from build123d import *
from build123d.topology import SkipClean

# Parameters (mm, degrees)
BOSS_EXTRUDE1_DEPTH     = 1.4
BOSS_EXTRUDE2_DEPTH     = 0.7
SKETCH3_W               = 2
SKETCH3_H               = 1
SKETCH3_R               = 2.5
BOSS_EXTRUDE3_DEPTH     = 0.6
SKETCH4_R               = 2
SKETCH4_R_2             = 0.75
SKETCH4_W               = 2
SKETCH4_H               = 1
BOSS_EXTRUDE4_DEPTH     = 1.3
BOSS_EXTRUDE6_REACH     = 14
CHAMFER1_SIZE           = 2
SKETCH7_W               = 12.5
SKETCH7_H               = 6.503126956
BOSS_EXTRUDE7_DEPTH     = 7.75
SKETCH8_W               = 12.5
SKETCH8_H               = 7.5
BOSS_EXTRUDE8_DEPTH     = 10
FILLET1_R               = 3
SKETCH9_W               = 11
SKETCH9_H               = 1.9
BOSS_EXTRUDE9_DEPTH     = 3.003289
BOSS_EXTRUDE10_START    = -0.75
SKETCH10_R              = 0.75
SKETCH10_R_2            = 2
SKETCH10_W              = 2
SKETCH10_H              = 1
BOSS_EXTRUDE10_DEPTH    = 0.75
SKETCH11_R              = 2
BOSS_EXTRUDE11_DEPTH    = 2.5
FILLET2_SIZE            = 2.5
FILLET2_SIZE_2          = 1
CUT_EXTRUDE1_DEPTH      = 32.401632123
CUT_EXTRUDE1_DEPTH_BACK = 32.401632123
SKETCH12_R              = 0.75
CUT_EXTRUDE2_REACH      = 34.731
SKETCH13_W              = 2.1
SKETCH13_H              = 1


with BuildPart() as part:
    # Sketch1 → Boss-Extrude1 (new body)
    with BuildSketch(Plane.XY):
        with BuildLine():
            Line((-5.5, 5.809475019), (-5.5, -2.5))
            Line((-5.5, -2.5), (-2.5, -5.5))
            Line((-2.5, -5.5), (2.5, -5.5))
            Line((2.5, -5.5), (5.5, -2.5))
            Line((5.5, -2.5), (5.5, 5.809475019))
            ThreePointArc((5.5, 5.809475019), (0, -8), (-5.5, 5.809475019))
        make_face()
    extrude(amount=BOSS_EXTRUDE1_DEPTH)

    # Sketch2 → Boss-Extrude2 (add)
    with BuildSketch(Plane.XY.offset(1.4)):
        with BuildLine():
            Line((-1, -5.5), (-1, -6.5))
            Line((-1, -6.5), (1, -6.5))
            Line((1, -6.5), (1, -5.5))
            Line((1, -5.5), (2.5, -5.5))
            Line((2.5, -5.5), (5.5, -2.5))
            Line((5.5, -2.5), (5.5, 5.809475019))
            ThreePointArc((5.5, 5.809475019), (0, -8), (-5.5, 5.809475019))
            Line((-5.5, 5.809475019), (-5.5, -2.5))
            Line((-5.5, -2.5), (-2.5, -5.5))
            Line((-2.5, -5.5), (-1, -5.5))
        make_face()
    extrude(amount=BOSS_EXTRUDE2_DEPTH)

    # Sketch3 → Boss-Extrude3 (add)
    with BuildSketch(Plane.XY.offset(2.1)):
        with BuildLine():
            Line((-5.5, 6.5), (-5.5, 5.809475019))
            ThreePointArc((-5.5, 5.809475019), (0, -8), (5.5, 5.809475019))
            Line((5.5, 5.809475019), (5.5, 6.5))
            Line((5.5, 6.5), (-5.5, 6.5))
        make_face()
        with Locations((0, -6)):
            Rectangle(SKETCH3_W, SKETCH3_H, mode=Mode.SUBTRACT)
        Circle(SKETCH3_R, mode=Mode.SUBTRACT)
        with BuildLine():
            ThreePointArc((-3.499999999, 5.5), (-4.249999999, 4.75), (-4.999999999, 5.5))
            ThreePointArc((-4.999999999, 5.5), (-4.249999999, 6.25), (-3.499999999, 5.5))
        make_face(mode=Mode.SUBTRACT)
        with BuildLine():
            ThreePointArc((5.000000001, 5.5), (4.250000001, 4.75), (3.500000001, 5.5))
            ThreePointArc((3.500000001, 5.5), (4.250000001, 6.25), (5.000000001, 5.5))
        make_face(mode=Mode.SUBTRACT)
    extrude(amount=BOSS_EXTRUDE3_DEPTH)

    # Sketch4 → Boss-Extrude4 (add)
    with SkipClean():  # the faces are left unmerged after this step: merging them gives an invalid solid
        with BuildSketch(Plane.XY.offset(2.7)):
            with BuildLine():
                Line((-5.5, 5.809475019), (-5.5, 6.5))
                Line((-5.5, 6.5), (5.5, 6.5))
                Line((5.5, 6.5), (5.5, 5.809475019))
                ThreePointArc((5.5, 5.809475019), (0, -8), (-5.5, 5.809475019))
            make_face()
            Circle(SKETCH4_R, mode=Mode.SUBTRACT)
            with Locations((-4.249999999, 5.5)):
                Circle(SKETCH4_R_2, mode=Mode.SUBTRACT)
            with Locations((4.250000001, 5.5)):
                Circle(SKETCH4_R_2, mode=Mode.SUBTRACT)
            with Locations((0, -6)):
                Rectangle(SKETCH4_W, SKETCH4_H, mode=Mode.SUBTRACT)
        extrude(amount=BOSS_EXTRUDE4_DEPTH)

    # Boss-Extrude6: up to this face of the body (flat: up to its plane)
    boss_extrude6_end = Plane(part.part.faces().sort_by_distance((0, -7.784071771, 4))[0])
    # Sketch5 → Boss-Extrude6 (add, up to the picked face)
    with BuildSketch(Plane.XY, mode=Mode.PRIVATE) as boss_extrude6_sk1:
        with BuildLine():
            Line((-6.25, 4.993746089), (-6.25, 18))
            Line((-6.25, 18), (6.25, 18))
            Line((6.25, 18), (6.25, 4.993746089))
            ThreePointArc((6.25, 4.993746089), (5.88914072, 5.414611858), (5.5, 5.809475019))
            Line((5.5, 5.809475019), (5.5, 6.5))
            Line((5.5, 6.5), (4.249999999, 8.5))
            ThreePointArc((4.249999999, 8.5), (0, 9.503288904), (-4.249999999, 8.5))
            Line((-4.249999999, 8.5), (-5.5, 6.5))
            Line((-5.5, 6.5), (-5.5, 5.809475019))
            ThreePointArc((-5.5, 5.809475019), (-5.88914072, 5.414611858), (-6.25, 4.993746089))
        make_face()
    boss_extrude6_tool1 = split(extrude(boss_extrude6_sk1.sketch, amount=BOSS_EXTRUDE6_REACH, mode=Mode.PRIVATE), bisect_by=boss_extrude6_end, keep=Keep.BOTH, mode=Mode.PRIVATE)
    add(boss_extrude6_tool1.solids().sort_by(Axis((0, 13.103061, 0), (0, 0, 1)))[0])

    # Chamfer1
    chamfer1_edges = [part.edges().sort_by_distance(p)[0] for p in [
        (0, 9.503288904, 0),
    ]]
    chamfer(chamfer1_edges, length=CHAMFER1_SIZE)

    # Sketch7 → Boss-Extrude7 (add)
    with BuildSketch(Plane(origin=(0, 0, 0), x_dir=(-1, 0, 0), z_dir=(0, 0, -1))):
        with Locations((0, 14.748436522)):
            Rectangle(SKETCH7_W, SKETCH7_H)
    extrude(amount=BOSS_EXTRUDE7_DEPTH)

    # Sketch8 → Boss-Extrude8 (add)
    with SkipClean():  # the faces are left unmerged after this step: merging them gives an invalid solid
        with BuildSketch(Plane(origin=(0, 18, 0), x_dir=(1, 0, 0), z_dir=(0, 1, 0))):
            with Locations((0, 4)):
                Rectangle(SKETCH8_W, SKETCH8_H)
        extrude(amount=BOSS_EXTRUDE8_DEPTH)

    # Fillet1
    # the kernel refuses this fillet: 3 mm, written as the material it adds along each edge
    with BuildSketch(Plane(origin=(-6.25, 18, -0.25), x_dir=(0, 0, 1), z_dir=(1, 0, 0))) as fillet1_piece_1:
        with BuildLine():
            CenterArc((FILLET1_R, -FILLET1_R), FILLET1_R, 90, 90)
            Line((0, -FILLET1_R), (0, 0))
            Line((0, 0), (FILLET1_R, 0))
        make_face()
    extrude(amount=12.5)

    # Sketch9 → Boss-Extrude9 (add)
    with BuildSketch(Plane(origin=(0, 6.5, 0), x_dir=(1, 0, 0), z_dir=(0, 1, 0))):
        with Locations((0, -3.05)):
            Rectangle(SKETCH9_W, SKETCH9_H)
    extrude(amount=BOSS_EXTRUDE9_DEPTH)

    # Sketch10 → Boss-Extrude10 (add)
    with SkipClean():  # the faces are left unmerged after this step: merging them gives an invalid solid
        with BuildSketch(Plane.XY.offset(4).offset(BOSS_EXTRUDE10_START)):
            with Locations((4.250000001, 5.5)):
                Circle(SKETCH10_R)
            with Locations((-4.249999999, 5.5)):
                Circle(SKETCH10_R)
            Circle(SKETCH10_R_2)
            with Locations((0, -6)):
                Rectangle(SKETCH10_W, SKETCH10_H)
        extrude(amount=BOSS_EXTRUDE10_DEPTH)
    add(part.part.scale(1), mode=Mode.REPLACE)  # the faces are merged on a copy

    # Sketch11 → Boss-Extrude11 (add)
    with BuildSketch(Plane(origin=(0, 0, -7.75), x_dir=(-1, 0, 0), z_dir=(0, 0, -1))):
        with Locations(Location((0, 15.622654783, 0), (0, 0, 180))):
            Circle(SKETCH11_R)
        with Locations(Location((0, 23.874218261, 0), (0, 0, 180))):
            Circle(SKETCH11_R)
    extrude(amount=BOSS_EXTRUDE11_DEPTH)

    # Fillet2
    # an asymmetric fillet: 2.5, 1 mm, written as the material it takes off along each edge
    with BuildSketch(Plane(origin=(0, 15.622654783, -10.25), x_dir=(1, 0, 0), z_dir=(0, 1, 0))) as fillet2_piece_1:
        with BuildLine():
            Bezier((2, -FILLET2_SIZE), (2, 0), (2 - FILLET2_SIZE_2, 0), weights=[1, 0.707106781, 1])
            Line((2 - FILLET2_SIZE_2, 0), (2, 0))
            Line((2, 0), (2, -FILLET2_SIZE))
        make_face()
    revolve(axis=Axis((0, 15.622654783, -10.25), (0, 0, -1)), mode=Mode.SUBTRACT)
    with BuildSketch(Plane(origin=(0, 23.874218261, -10.25), x_dir=(1, 0, 0), z_dir=(0, 1, 0))) as fillet2_piece_2:
        with BuildLine():
            Bezier((2, -FILLET2_SIZE), (2, 0), (2 - FILLET2_SIZE_2, 0), weights=[1, 0.707106781, 1])
            Line((2 - FILLET2_SIZE_2, 0), (2, 0))
            Line((2, 0), (2, -FILLET2_SIZE))
        make_face()
    revolve(axis=Axis((0, 23.874218261, -10.25), (0, 0, -1)), mode=Mode.SUBTRACT)

    # Sketch12 → Cut-Extrude1 (cut, two sides: drawn at the far end of the back side and taken through both)
    with BuildSketch(Plane(origin=(0, 0, -7.75), x_dir=(-1, 0, 0), z_dir=(0, 0, -1)).offset(-CUT_EXTRUDE1_DEPTH_BACK)):
        with Locations((-4.25, 15.7375)):
            Circle(SKETCH12_R)
        with Locations((-4.25, 23.9125)):
            Circle(SKETCH12_R)
        with Locations((4.25, 23.9125)):
            Circle(SKETCH12_R)
        with Locations((4.25, 15.7375)):
            Circle(SKETCH12_R)
    extrude(amount=CUT_EXTRUDE1_DEPTH + CUT_EXTRUDE1_DEPTH_BACK, mode=Mode.SUBTRACT)

    # Cut-Extrude2: up to this face of the body (flat: up to its plane)
    cut_extrude2_end = Plane(part.part.faces().sort_by_distance((-5.5, 2, 1.05))[0])
    # Sketch13 → Cut-Extrude2 (cut, up to the picked face)
    with BuildSketch(Plane.ZY.offset(-5.5), mode=Mode.PRIVATE) as cut_extrude2_sk1:
        with Locations((1.05, 7)):
            Rectangle(SKETCH13_W, SKETCH13_H)
    cut_extrude2_tool1 = split(extrude(cut_extrude2_sk1.sketch, amount=CUT_EXTRUDE2_REACH, mode=Mode.PRIVATE), bisect_by=cut_extrude2_end, keep=Keep.BOTH, mode=Mode.PRIVATE)
    add(cut_extrude2_tool1.solids().sort_by(Axis((5.5, 7, 1.05), (-1, 0, 0)))[0], mode=Mode.SUBTRACT)


solid = part.part
Model file for the job. Use its own axes, mm. A direction names the side the tool comes from. Coordinates: 2 decimals unless noted, no trailing zeros. Write each loop counter-clockwise with the first axis right and the second up, starting at its lowest first coordinate (ties: lowest second). Pieces come first, ordered by that corner, then holes. Notation, with made-up numbers: (-3, 2) -> (26, 2) arc R30 cw to (26, 36) -> close; hole circle Ø8 at (-33, -1.5). An arc over 180 degrees is marked (long way). One line per item, written item: value. Start each with the question number.
1) Probe probe 1 along Y at (x, z) = (0, 2.55); probe 2 along Y at (x, z) = (4.25, -6); probe 3 along X at (y, z) = (5.5, 2.9). List the from-to ranges inside material, lowest first.
2) Flat gauge pins, fed straight in: pin 1 Ø0.5 at (x, z) = (-5.5, 0.5) entering from -Y; pin 2 Ø1.7 at (x, y) = (-4.25, 23.91) entering from -Z; pin 3 Ø6 at (x, z) = (2, -5) entering from -Y; pin 4 Ø1.5 at (y, z) = (9.5, -1.5) entering from -X. Where does each tip first touch, or does it go through?
3) Which spindle directions (+Z, -Z, +X, -X, +Y, -Y) get a long thin tool onto all of the face, cutting with end or side? Do faces 5 (the face through (-6, 0, 0)), 6 (the face through (0, -6, 3.25)), 7 (the face through (0.1, 10.3, 1.2)). Say none if no direction does.
4) Slice it at B-B on z = -1.5. Write the cut outline in (x, y), then the cut area to 3 significant figures.
5) Slice it at C-C on y = 20. Write the cut outline in (x, z).
6) Pull direction Y, two halves, no side cores. Call faces 1 (the face through (-0.09, 18.86, 0.65)), 2 (the face through (4, 8.9, 0.8)), 3 (the face through (0, 0, 3.25)), 4 (the face through (0, 11.497, -4)): +Y half, -Y half, draft (parallel to the pull), parting line (faces both ways), or undercut.
7) Slice it at A-A on y = 0. Write the cut outline in (x, z).
Answers follow:
1. probe 1: -8 to -6.5, -5.5 to -2.5, 2.5 to 18.01
1. probe 2: 11.5 to 14.99, 16.49 to 23.16, 24.66 to 28
1. probe 3: -6.25 to -5, -3.5 to 3.5, 5 to 6.25
2. pin 1: y = -6.04
2. pin 2: z = -7.75
2. pin 3: y = 11.5
2. pin 4: through
3. face 5: -Z, +X, -X, -Y
3. face 6: none
3. face 7: -Z
4. outline: (-6.25, 11.5) -> (6.25, 11.5) -> (6.25, 28) -> (-6.25, 28) -> close; hole circle Ø1.5 at (-4.25, 15.74); hole circle Ø1.5 at (-4.25, 23.91); hole circle Ø1.5 at (4.25, 15.74); hole circle Ø1.5 at (4.25, 23.91)
4. area: 199 mm2
5. outline: (-6.25, -7.75) -> (6.25, -7.75) -> (6.25, -0.08) -> (-6.25, -0.08) -> close
6. face 1: +Y half
6. face 2: undercut
6. face 3: undercut
6. face 4: -Y half
7. outline: (-8, 0) -> (-5.5, 0) -> (-5.5, 2.1) -> (-2.5, 2.1) -> (-2.5, 2.7) -> (-2, 2.7) -> (-2, 3.25) -> (2, 3.25) -> (2, 2.7) -> (2.5, 2.7) -> (2.5, 2.1) -> (5.5, 2.1) -> (5.5, 0) -> (8, 0) -> (8, 4) -> (-8, 4) -> close
